```python
from build123d import *

# Parameters (mm, degrees)
BOSS_EXTRUDE1_DEPTH = 5
SKETCH4_R           = 1.5
BOSS_EXTRUDE3_DEPTH = 20
CUT_EXTRUDE2_START  = 2
CUT_EXTRUDE2_DEPTH  = 1
CUT_EXTRUDE4_START  = -2
CUT_EXTRUDE4_DEPTH  = 1


with BuildPart() as part:
    # Sketch1 → Boss-Extrude1 (new, symmetric)
    with BuildSketch(Plane.XY):
        with BuildLine():
            Line((10, 2.25), (-10, 2.25))
            ThreePointArc((-10, 2.25), (-12.25, 0), (-10, -2.25))
            Line((-10, -2.25), (10, -2.25))
            ThreePointArc((10, -2.25), (12.25, 0), (10, 2.25))
        make_face()
    extrude(amount=BOSS_EXTRUDE1_DEPTH, both=True)

    # Sketch4 → Boss-Extrude3 (add)
    with BuildSketch(Plane.XY.offset(5)):
        Circle(SKETCH4_R)
    extrude(amount=BOSS_EXTRUDE3_DEPTH)

    # Sketch1<4> → Cut-Extrude2 (cut, symmetric)
    with BuildSketch(Plane.XY.offset(CUT_EXTRUDE2_START)):
        with BuildLine():
            Line((0, 2.25), (-10, 2.25))
            ThreePointArc((-10, 2.25), (-12.25, 0), (-10, -2.25))
            Line((-10, -2.25), (0, -2.25))
            Line((0, -2.25), (10, -2.25))
            ThreePointArc((10, -2.25), (12.25, 0), (10, 2.25))
            Line((10, 2.25), (0, 2.25))
        make_face()
        with BuildLine():
            Line((0, 1.25), (-10, 1.25))
            ThreePointArc((-10, 1.25), (-11.25, 0), (-10, -1.25))
            Line((-10, -1.25), (0, -1.25))
            Line((0, -1.25), (10, -1.25))
            ThreePointArc((10, -1.25), (11.25, 0), (10, 1.25))
            Line((10, 1.25), (0, 1.25))
        make_face(mode=Mode.SUBTRACT)
    extrude(amount=CUT_EXTRUDE2_DEPTH, both=True, mode=Mode.SUBTRACT)

    # Sketch1<6> → Cut-Extrude4 (cut, symmetric)
    with BuildSketch(Plane.XY.offset(CUT_EXTRUDE4_START)):
        with BuildLine():
            Line((0, 2.25), (-10, 2.25))
            ThreePointArc((-10, 2.25), (-12.25, 0), (-10, -2.25))
            Line((-10, -2.25), (0, -2.25))
            Line((0, -2.25), (10, -2.25))
            ThreePointArc((10, -2.25), (12.25, 0), (10, 2.25))
            Line((10, 2.25), (0, 2.25))
        make_face()
        with BuildLine():
            Line((0, 1.25), (-10, 1.25))
            ThreePointArc((-10, 1.25), (-11.25, 0), (-10, -1.25))
            Line((-10, -1.25), (0, -1.25))
            Line((0, -1.25), (10, -1.25))
            ThreePointArc((10, -1.25), (11.25, 0), (10, 1.25))
            Line((10, 1.25), (0, 1.25))
        make_face(mode=Mode.SUBTRACT)
    extrude(amount=CUT_EXTRUDE4_DEPTH, both=True, mode=Mode.SUBTRACT)


solid = part.part
```
For this review, take the finished solid that the model builds, in its own axes (mm). A direction names the side the tool comes from. Give positions to 0.01 mm unless a question says otherwise; leave off trailing zeros. Write each loop counter-clockwise with the first axis right and the second up, starting at its lowest first coordinate (ties: lowest second). Pieces come first, ordered by that corner, then holes. Notation, with made-up numbers: M 56,-3 L 109,-3 A8 ccw 109,6 Z; hole C 42,37 d7. An arc over 180 degrees is marked long. One line per item, written item: value.
1) Take a section at A-A, the plane x = -2. Write out the cut boundary in (y, z).
Results are:
outline: M -2.25,-5 L 2.25,-5 L 2.25,-3 L 1.25,-3 L 1.25,-1 L 2.25,-1 L 2.25,1 L 1.25,1 L 1.25,3 L 2.25,3 L 2.25,5 L -2.25,5 L -2.25,3 L -1.25,3 L -1.25,1 L -2.25,1 L -2.25,-1 L -1.25,-1 L -1.25,-3 L -2.25,-3 Z
2) Take a section at B-B, the plane y = 0. Write out the cut boundary in (x, z), then the cut area to 3 significant figures.
Results are:
outline: M -12.25,-5 L 12.25,-5 L 12.25,-3 L 11.25,-3 L 11.25,-1 L 12.25,-1 L 12.25,1 L 11.25,1 L 11.25,3 L 12.25,3 L 12.25,5 L 1.5,5 L 1.5,25 L -1.5,25 L -1.5,5 L -12.25,5 L -12.25,3 L -11.25,3 L -11.25,1 L -12.25,1 L -12.25,-1 L -11.25,-1 L -11.25,-3 L -12.25,-3 Z
area: 297 mm²
3) Take a section at C-C, the plane z = 4.5. Write out the cut boundary in (x, y).
Results are:
outline: M -10,-2.25 L 10,-2.25 A2.25 ccw 10,2.25 L -10,2.25 A2.25 ccw Z
4) The part is to be moulded in two halves that separate along Z. For faces 1 (the flat face through (0, 0, -5)), 2 (the flat face through (0, -2.25, 0)), 3 (the flat face through (-0.2, -1.5, 1)), say which applies: +Z half, -Z half, draft (parallel to the pull), parting line (faces both ways), or undercut.
Results are:
face 1: -Z half
face 2: draft
face 3: undercut
5) For faces 4 (the cylindrical face through (-11.25, 0.03, -1.99)), 5 (the cylindrical face through (-12.25, 0.05, -3.99)), 6 (the cylindrical face through (11.25, -0.03, -1.99)), 7 (the flat face through (0, -1.25, -2)), list the 3-axis set-ups (+Z, -Z, +X, -X, +Y, -Y) from which the entire face can be reached by the end or side of a thin tool; tool diameter is ignored.
Results are:
face 4: -X
face 5: +Z, -Z, -X
face 6: +X
face 7: +X, -X, -Y
6) For P1, Ø1.6, axis at x = -3, z = -2, coming from the +Y side; P2, Ø8, axis at x = 5, z = 12.5, coming from the +Y side; P3, Ø1.5, axis at y = -1, z = 21.5, coming from the +X side, all flat-tipped, find the tip position at first contact; note any pin that passes through.
Results are:
P1: stops at y = 1.25
P2: stops at y = 1.12
P3: stops at x = 1.48
7) Take a section at D-D, the plane x = 0.5. Write out the cut boundary in (y, z), then the cut area to 3 significant figures.
Results are:
outline: M -2.25,-5 L 2.25,-5 L 2.25,-3 L 1.25,-3 L 1.25,-1 L 2.25,-1 L 2.25,1 L 1.25,1 L 1.25,3 L 2.25,3 L 2.25,5 L 1.41,5 L 1.41,25 L -1.41,25 L -1.41,5 L -2.25,5 L -2.25,3 L -1.25,3 L -1.25,1 L -2.25,1 L -2.25,-1 L -1.25,-1 L -1.25,-3 L -2.25,-3 Z
area: 93.6 mm²
8) For line 1 (Z direction, x = 7.25, y = 2.05); line 2 (Z direction, x = -4.5, y = 0.2); line 3 (X direction, y = 1.65, z = 0.25), list the stretches that pass through material, from the lowest coordinate up. Write a range as from..to.
Results are:
line 1: z = -5..-3, -1..1, 3..5
line 2: z = -5..5
line 3: x = -11.53..11.53
